Part model, mm, in its own coordinate system. A direction names the side the tool comes from. Coordinates: 2 decimals unless noted, no trailing zeros. Write each loop counter-clockwise with the first axis right and the second up, starting at its lowest first coordinate (ties: lowest second). Pieces come first, ordered by that corner, then holes. Notation, with made-up numbers: (-13.5, 88.25) -> (8.5, 88.25) arc R24 ccw to (8.5, 126.25) -> close; hole circle Ø6 at (17, 46). An arc over 180 degrees is marked (long way). Write item = value, one per line. Start each with the question number.
Q1. Band-saw the part on A-A, the plane x = -289.5. List the corners of the cut face in (y, z), plus the area to 3 significant figures.
Q2. Probe line 1 (Y direction, x = -289, z = 7.5); line 2 (Y direction, x = -150.5, z = 1). List the from-to ranges inside material, lowest first.
Q3. Tool access for faces 1 (the flat face through (-7, 26, 2)), 2 (the flat face through (-7, 26, 0)): list every direction of +Z, -Z, +X, -X, +Y, -Y with a clear straight run to the whole face (end or side of a thin tool).
Q4. Band-saw the part on B-B, the plane z = 13.5. List the corners of the cut face in (x, y), plus the area to 3 significant figures.
Q5. Pin check, flat tips, straight feed: P1, Ø3, axis at x = -128, z = 14.5, coming from the +Y side; P2, Ø12, axis at y = 40.5, z = 13, coming from the +X side; P3, Ø1, axis at x = -245, z = 1, coming from the +Y side; P4, Ø20.5, axis at x = -226.5, y = 22, coming from the +Z side. Stop position of each tip, or through.
Autodesk Inventor part; units mm, degrees
ref_plane "YZ Plane" through (0, 0, 0) normal (1, 0, 0) x (0, 1, 0)
ref_plane "XZ Plane" through (0, 0, 0) normal (0, 1, 0) x (-1, 0, 0)
ref_plane "XY Plane" through (0, 0, 0) normal (0, 0, 1) x (1, 0, 0)
sketch "Sketch1" plane through (0, 0, 0) normal (0, 0, 1) x (1, 0, 0)
  line L0 (-490, 46) -> (490, 46)
  line L1 (490, 46) -> (490, 0)
  line L2 (490, 0) -> (-490, 0)
  line L3 (-490, 0) -> (-490, 46)
  point P0 (0, 0)
  point P1 (0, 0)
  dimension "d0" = 980
  dimension "d1" = 46
extrude "Plate1" add sketch "Sketch1" along normal blind 2
sketch "Sketch2" plane through (490, 2, 0) normal (0, -1, 0) x (1, 0, 0)
  line L0 (-980, 0) -> (0, 0)
  line L1 (0, 0) -> (0, 20)
  line L2 (0, 20) -> (-980, 20)
  line L3 (-980, 20) -> (-980, 0)
edge flange "Flange1" height 20 angle 90 thickness 2 bend radius 2.75 thickness toward (0, -1, 0) relief round relief width 2 relief depth 1 edges at (0, 0, 2) wall of the first edge with corners at (-490, 2, 0) (490, 2, 0) (490, 2, 20) (-490, 2, 20)
bend "Bend1"
corner "Corner1"
sketch "Sketch5" plane through (0, 0, 0) normal (0, 0, -1) x (-1, 0, 0)
  line L0 (490, 46) -> (-490, 46)
  line L1 (490, 0) -> (-490, 0)
  circle A0 centre (0, 46) radius 35
  line L2 (243.95, 46) -> (246.05, 46)
  line L3 (246.05, 46) -> (246.05, 29)
  line L4 (246.05, 29) -> (243.95, 29)
  line L5 (243.95, 29) -> (243.95, 46)
  line L6 (-243.95, 46) -> (-246.05, 46)
  line L7 (-246.05, 46) -> (-246.05, 29)
  line L8 (-246.05, 29) -> (-243.95, 29)
  line L9 (-243.95, 29) -> (-243.95, 46)
  line L10 (0, 46) -> (0, 0) construction
  line L11 (490, 0) -> (490, 46)
  line L12 (-490, 0) -> (-490, 46)
  circle A1 centre (-490, 46) radius 35
  circle A2 centre (490, 46) radius 35
  point P0 (0, 0)
  point P1 (245, 29)
  point P2 (-245, 29)
  point P3 (246.05, 46)
  point P4 (-35, 46)
  point P5 (35, 46)
  point P6 (-246.05, 46)
  point P7 (455, 46)
  point P8 (490, 11)
  point P9 (-490, 11)
  point P10 (-455, 46)
  dimension "d45" = 70
  dimension "d48" = 2.1
  dimension "d49" = 490
  dimension "d51" = 29
  dimension "d52" = 17
extrude "Extrusion1" cut sketch "Sketch5" against normal through all contours L3 L4 L5 L0 | L0 L11 A2 | L9 L8 L7 L0 | L12 L0 A1 picked at (473.6046, 29.6046) picked at (-466.9592, 43.4039)
sketch "Sketch9" plane through (0, 0, 2) normal (0, 0, 1) x (1, 0, 0)
  line L0 (448.2795, 24.3045) -> (448.2795, 12.3045) construction
  line L1 (448.2795, 12.3045) -> (248.2795, 12.3045) construction
  line L2 (248.2795, 12.3045) -> (248.2795, 24.3045) construction
  line L3 (248.2795, 24.3045) -> (448.2795, 24.3045) construction
  line L4 (-490, 46) -> (490, 46)
  point P0 (0, 0)
  point P1 (1.05, 68)
  point P2 (490, 46)
  point P3 (-490, 46)
  dimension "d40" = 200
  dimension "d41" = 12
mark "Mark2"
equation "\"d2\" = Thickness"
equation "\"d3\" = BendReliefWidth"
equation "\"d4\" = BendReliefDepth"
equation "\"d5\" = MinimumRemnant"
equation "\"d6\" = TransitionRadius"
equation "\"d9\" = BendRadius"
equation "\"d10\" = CornerReliefSize"
equation "\"d11\" = GapSize"
equation "\"d12\" = JacobiRadiusSize"
equation "\"BendReliefWidth\" = Thickness"
equation "\"BendReliefDepth\" = 0.5 * Thickness"
equation "\"CornerReliefSize\" = 4 * Thickness"
equation "\"MinimumRemnant\" = 2 * Thickness"
equation "\"TransitionRadius\" = BendRadius"
equation "\"JacobiRadiusSize\" = BendRadius"
equation "\"GapSize\" = Thickness"
properties part number "MSC 307 stringer BOARD  ##" material "Stainless Steel"
Ans:
q1.outline = (0, 4.75) arc R4.75 ccw to (4.75, 0) -> (46, 0) -> (46, 2) -> (4.75, 2) arc R2.75 cw to (2, 4.75) -> (2, 20) -> (0, 20) -> close
q1.area = 125 mm2
q2.line_1 = 0 to 2
q2.line_2 = 1.83 to 46
q3.face_1 = +Z, +X, -X, +Y
q3.face_2 = -Z, +X, -X, +Y, -Y
q4.outline = (-490, 0) -> (490, 0) -> (490, 2) -> (-490, 2) -> close
q4.area = 1,960 mm2
q5.P1 = 2
q5.P2 = through
q5.P3 = 29
q5.P4 = 2
